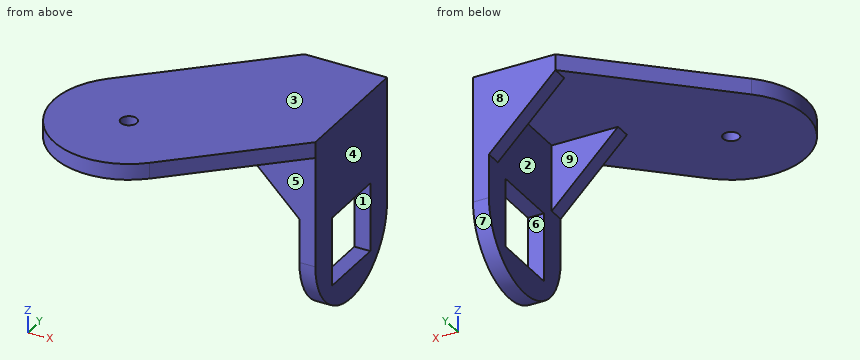
```python
from build123d import *

# Parameters (mm, degrees)
SKETCH2_R           = 5
BOSS_EXTRUDE1_DEPTH = 10
SKETCH5_W           = 43
SKETCH5_H           = 43
BOSS_EXTRUDE3_DEPTH = 10
BOSS_EXTRUDE4_DEPTH = 10


with BuildPart() as part:
    # Sketch2 → Boss-Extrude1 (new body)
    with BuildSketch(Plane.XY):
        with BuildLine():
            Line((790.019647556, 783.678215824), (709.10700943, 708.225960112))
            ThreePointArc((709.10700943, 708.225960112), (706.787308377, 641.798413213), (773.214855276, 639.47871216))
            Line((773.214855276, 639.47871216), (841.59626274, 703.245406232))
            Line((841.59626274, 703.245406232), (841.59626274, 783.678215824))
            Line((841.59626274, 783.678215824), (790.019647556, 783.678215824))
        make_face()
        with Locations((741.160932353, 673.852336136)):
            Circle(SKETCH2_R, mode=Mode.SUBTRACT)
    extrude(amount=BOSS_EXTRUDE1_DEPTH)

    # Sketch5 → Boss-Extrude3 (add)
    with BuildSketch(Plane(origin=(841.59626274, 0, 0), x_dir=(0, 0, -1), z_dir=(1, 0, 0))):
        with BuildLine():
            Line((69, 783.678215824), (0, 783.678215824))
            Line((0, 783.678215824), (0, 703.245406232))
            Line((0, 703.245406232), (69, 703.245406232))
            ThreePointArc((69, 703.245406232), (109.216404796, 743.461811028), (69, 783.678215824))
        make_face()
        with Locations((69, 743.461811028)):
            Rectangle(SKETCH5_W, SKETCH5_H, mode=Mode.SUBTRACT)
    extrude(amount=-BOSS_EXTRUDE3_DEPTH)

    # Sketch6 → Boss-Extrude4 (add)
    with BuildSketch(Plane(origin=(0, 783.678215824, 0), x_dir=(1, 0, 0), z_dir=(0, 1, 0))):
        Polygon((790.019647556, 0), (831.59626274, 41.576615184), (831.59626274, 0), align=None)
    boss_extrude4 = extrude(amount=-BOSS_EXTRUDE4_DEPTH)

    # Mirror1: Boss-Extrude4 across plane
    add(boss_extrude4.mirror(Plane.ZX.offset(743.461811028)))


solid = part.part
```
Here's how the part is built. I have some questions about the finished solid (model axes, mm). Face numbers are marked on the shaded views. A direction names the side the tool comes from. Coordinates: 2 decimals unless noted, no trailing zeros. Loops run counter-clockwise (first coordinate to the right, second up) from the corner with the lowest first, then second, coordinate; pieces in that order, holes last. Notation, with made-up numbers: M 3,68 L 15,68 A19 cw 15,102 Z; hole C 3.25,-11.5 d2. An arc over 180 degrees is marked long. One line per item, written item: value.
1. Imagine slicing it at B-B (y = 730). List the corners of the cut face in (x, z) for me, and give its area (3 significant figures).
Geometry says:
outline: M 732.46,0 L 831.6,0 L 831.6,-47.5 L 841.6,-47.5 L 841.6,10 L 732.46,10 Z; M 831.6,-106.9 L 841.6,-106.9 L 841.6,-90.5 L 831.6,-90.5 Z
area: 1,730 mm2
2. Will these pins go through, and if not, where does the flat tip stop? pin 1 Ø3 at (x, y) = (837, 739) entering from -Z; pin 2 Ø13 at (x, y) = (741.16, 673.85) entering from -Z; pin 3 Ø1 at (y, z) = (723.5, -4.5) entering from -X.
Geometry says:
pin 1: stops at z = -109.11
pin 2: stops at z = 0
pin 3: stops at x = 831.6
3. Imagine slicing it at A-A (z = -75.5). List the corners of the cut face in (x, y) for me, and give its area (3 significant figures).
Geometry says:
outline: M 831.6,703.77 L 841.6,703.77 L 841.6,721.96 L 831.6,721.96 Z; M 831.6,764.96 L 841.6,764.96 L 841.6,783.15 L 831.6,783.15 Z
area: 364 mm2
4. On a 3-axis mill with a long thin cutter (end or side, diameter ignored), from which of +Z, -Z, +X, -X, +Y, -Y can I reach the whole of each face in a straight line? I mean the marked faces 1, 2, 3, 4 and 5. Say none if no direction works.
Geometry says:
face 1: +X, -X
face 2: -Z, -X
face 3: +Z, +X, -X, +Y, -Y
face 4: +Z, -Z, +X, +Y, -Y
face 5: -Z, +X, -X, -Y
5. Please list where these lines run through material, in increasing order: probe 1 along Y at (x, z) = (823, -10.5); probe 2 along Z at (x, y) = (832.5, 695); probe 3 along X at (y, z) = (760, -7.5).
Geometry says:
probe 1: y = 703.25 to 713.25, 773.68 to 783.68
probe 2: z = 0 to 10
probe 3: x = 831.6 to 841.6
6. Imagine slicing it at D-D (z = -39). List the corners of the cut face in (x, y) for me.
Geometry says:
outline: M 829.02,703.25 L 841.6,703.25 L 841.6,783.68 L 829.02,783.68 L 829.02,773.68 L 831.6,773.68 L 831.6,713.25 L 829.02,713.25 Z
7. Imagine slicing it at C-C (x = 820.5). List the corners of the cut face in (y, z) for me, and give its area (3 significant figures).
Geometry says:
outline: M 683.57,0 L 703.25,0 L 703.25,-30.48 L 713.25,-30.48 L 713.25,0 L 773.68,0 L 773.68,-30.48 L 783.68,-30.48 L 783.68,10 L 683.57,10 Z
area: 1,610 mm2
8. Thinking about a two-plate mould opening in Y: for the marked faces 6, 7, 8 and 9, which applies, +Y half, -Y half, draft (parallel to the pull), parting line (faces both ways), or undercut?
Geometry says:
face 6: undercut
face 7: parting line
face 8: +Y half
face 9: undercut
